```python
from build123d import *

# Parameters (mm, degrees)
F0_W     = 72
F0_H     = 20
F0_R     = 2
F0_R_2   = 5
F1_DEPTH = 10


with BuildPart() as f1:
    # F0 (on Front) → F1 (new body)
    with BuildSketch(Plane.XZ):
        with Locations((-36, -10)):
            Rectangle(F0_W, F0_H)
        with Locations((-44, -10)):
            Circle(F0_R, mode=Mode.SUBTRACT)
        with Locations((-36, -10)):
            Circle(F0_R_2, mode=Mode.SUBTRACT)
        with Locations((-28, -10)):
            Circle(F0_R, mode=Mode.SUBTRACT)
    extrude(amount=F1_DEPTH)


solid = f1.part
```
Could you check a few things on this model? Use its own coordinates, in mm. Give positions to 0.01 mm unless a question says otherwise; leave off trailing zeros. Loops run counter-clockwise (first coordinate to the right, second up) from the corner with the lowest first, then second, coordinate; pieces in that order, holes last. Notation, with made-up numbers: (41, 19.25) -> (48, 19.25) arc R34 cw to (48, 56.25) -> close; hole circle Ø6 at (55.5, 72). An arc over 180 degrees is marked (long way). Put each result on its own line as item: value.
(1) Imagine slicing it at B-B on y = -4.5. Write out the boundary of the cut face in (x, z), plus the area to 3 significant figures.
Computed:
outline: (-72, -20) -> (0, -20) -> (0, 0) -> (-72, 0) -> close; hole circle Ø4 at (-44, -10); hole circle Ø10 at (-36, -10); hole circle Ø4 at (-28, -10)
area: 1,340 mm^2
(2) Imagine slicing it at D-D on z = -13. Write out the boundary of the cut face in (x, y).
Computed:
outline: (-72, -10) -> (-40, -10) -> (-40, 0) -> (-72, 0) -> close; (-32, -10) -> (0, -10) -> (0, 0) -> (-32, 0) -> close
(3) Thinking about a two-plate mould opening in X: for faces 1 (the face through (-26.092, -4.93, -9.399)), 2 (the face through (0, -5, -10)), 3 (the face through (-37, -10, -3)), which applies, pulls with the +X half, pulls with the -X half, needs draft (parallel to the pull), parting line crosses it, or undercut?
Computed:
face 1: undercut
face 2: pulls with the +X half
face 3: needs draft
(4) Please list where these lines run through material, in increasing order: probe 1 along X at (y, z) = (-1.25, -8.5); probe 2 along Z at (x, y) = (-36, -2.25); probe 3 along Z at (x, y) = (-28.5, -9.25). Write a range as [from, to].
Computed:
probe 1: [-72, -45.32], [-42.68, -40.77], [-31.23, -29.32], [-26.68, 0]
probe 2: [-20, -15], [-5, 0]
probe 3: [-20, -11.94], [-8.06, 0]
(5) Imagine slicing it at C-C on z = -10. Write out the boundary of the cut face in (x, y).
Computed:
outline: (-72, -10) -> (-46, -10) -> (-46, 0) -> (-72, 0) -> close; (-42, -10) -> (-41, -10) -> (-41, 0) -> (-42, 0) -> close; (-31, -10) -> (-30, -10) -> (-30, 0) -> (-31, 0) -> close; (-26, -10) -> (0, -10) -> (0, 0) -> (-26, 0) -> close
(6) Imagine slicing it at A-A on x = -28. Write out the boundary of the cut face in (y, z).
Computed:
outline: (-10, -20) -> (0, -20) -> (0, -12) -> (-10, -12) -> close; (-10, -8) -> (0, -8) -> (0, 0) -> (-10, 0) -> close
